Geometry: final body of the model. Coordinates: model frame, mm. A direction names the side the tool comes from. Coordinates: 2 decimals unless noted, no trailing zeros. Order: outer loops, then holes, each group sorted by start corner. A loop starts at its lowest first (then second) coordinate and runs counter-clockwise, first axis right, second up. Notation, with made-up numbers: M -22.5,54.5 L 32.5,54.5 A19 cw 32.5,77.5 Z; hole C 8.25,83.25 d3. An arc over 180 degrees is marked long. Write item = value, one per line.
from build123d import *

# Parameters (mm, degrees)
EXTRUDE_1_DEPTH          = 10
CUT_EXTRUDE_1_DEPTH      = 24.452078799
CUT_EXTRUDE_1_DEPTH_BACK = 24.452078799
SKETCH_2_R               = 1.674991146


with BuildPart() as part:
    # ｽｹｯﾁ1 → ﾎﾞｽ - 押し出し1 (new body)
    with BuildSketch(Plane.XY):
        Polygon((-15, 0), (15, 0), (15, -5), (5, -5), (5, -20), (-5, -20), (-5, -5), (-15, -5), align=None)
    extrude(amount=EXTRUDE_1_DEPTH)

    # ｽｹｯﾁ2 → ｶｯﾄ - 押し出し1 (cut, two sides: drawn at the far end of the back side and taken through both)
    with BuildSketch(Plane.XZ.offset(5).offset(-CUT_EXTRUDE_1_DEPTH_BACK)):
        with Locations((-10, 5)):
            Circle(SKETCH_2_R)
        with Locations((10, 5)):
            Circle(SKETCH_2_R)
    extrude(amount=CUT_EXTRUDE_1_DEPTH + CUT_EXTRUDE_1_DEPTH_BACK, mode=Mode.SUBTRACT)


solid = part.part
1) Section D-D, the plane x = -6.25. Return loops of the section in (y, z), and give its area (3 significant figures).
Numbers:
outline = M -5,0 L 0,0 L 0,10 L -5,10 Z
area = 50.0 mm²
2) Mould query, pull axis Z, two halves, no side actions, for faces 4 (the face through (15, -2, 5)), 5 (the face through (0, -8, 0)), 6 (the face through (8.765, -2.465, 6.132)), 7 (the face through (0, -8, 10)). Classes: pulls with the +Z half, pulls with the -Z half, needs draft (parallel to the pull), parting line crosses it, or undercut.
Numbers:
face_4 = needs draft
face_5 = pulls with the -Z half
face_6 = undercut
face_7 = pulls with the +Z half
3) Line query: L1, parallel to X at y = -3.3, z = 5 (3 decimals); L2, parallel to Z at x = 10, y = -2.85 (3 decimals); L3, parallel to Y at x = 12.5, z = 5.5. Output: solid intervals per line, ascending.
Numbers:
L1 = -15 to -11.675, -8.325 to 8.325, 11.675 to 15
L2 = 0 to 3.325, 6.675 to 10
L3 = -5 to 0
4) Section C-C, the plane z = 1. Return loops of the section in (x, y), and give its area (3 significant figures).
Numbers:
outline = M -15,-5 L -5,-5 L -5,-20 L 5,-20 L 5,-5 L 15,-5 L 15,0 L -15,0 Z
area = 300 mm²
5) Set-up query: faces 1 (the face through (12, -5, 5)), 2 (the face through (0, -20, 5)), 3 (the face through (-5, -13, 5)). Return all of +Z, -Z, +X, -X, +Y, -Y with unobstructed straight access to the full face (end or side cutting, diameter ignored); none if empty.
Numbers:
face_1 = +Z, -Z, +X, -Y
face_2 = +Z, -Z, +X, -X, -Y
face_3 = +Z, -Z, -X, -Y
6) Pin query (flat end, axial travel): pin 1 (4.5 mm diameter, centred on x = -10, z = 5, fed in from -Y); pin 2 (6 mm diameter, centred on x = -5.5, y = -11.5, fed in from +Z); pin 3 (1 mm diameter, centred on x = 9, y = -6, fed in from -Z). Return the tip coordinate at first contact, or that it passes through.
Numbers:
pin_1 = -5
pin_2 = 10
pin_3 = through
7) Section B-B, the plane y = -4.5. Return loops of the section in (x, z) (3 decimals).
Numbers:
outline = M -15,0 L 15,0 L 15,10 L -15,10 Z; hole C -10,5 d3.35; hole C 10,5 d3.35
8) Section A-A, the plane x = 10. Return loops of the section in (y, z) (3 decimals), and give its area (4 significant figures).
Numbers:
outline = M -5,0 L 0,0 L 0,3.325 L -5,3.325 Z; M -5,6.675 L 0,6.675 L 0,10 L -5,10 Z
area = 33.25 mm²
